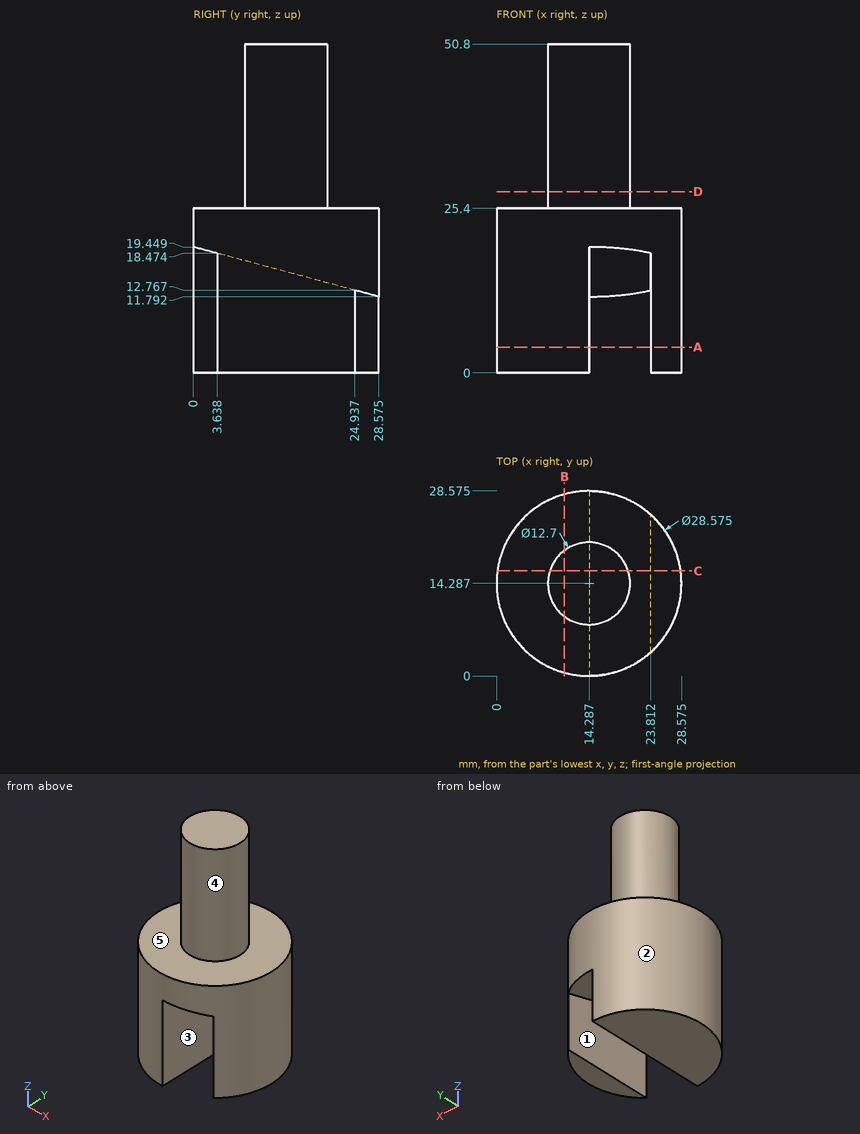
Geometry: see drawing. Coordinates: mm, zero at the bounding-box minimum. A direction names the side the tool comes from. Give positions to 0.01 mm unless a question says otherwise; leave off trailing zeros. Write each loop counter-clockwise with the first axis right and the second up, starting at its lowest first coordinate (ties: lowest second). Pieces come first, ordered by that corner, then holes. Notation, with made-up numbers: M 65,48 L 83,48 A16 ccw 83,68 Z; hole C -16.5,-21.5 d7. An arc over 180 degrees is marked long. Answer as a JSON object with one key per item and string values.
Q1. Cut plane C-C, the plane y = 16.25. Return the cut outline in (x, z) (1 decimal).
Geometry check:
{"outline": "M 0.1,0 L 14.3,0 L 14.3,15.1 L 23.8,15.1 L 23.8,0 L 28.4,0 L 28.4,25.4 L 20.3,25.4 L 20.3,50.8 L 8.2,50.8 L 8.2,25.4 L 0.1,25.4 Z"}
Q2. Access query for the marked faces 1 and 2. Directions: +Z, -Z, +X, -X, +Y, -Y. A direction counts if a zero-diameter tool reaches every point of the face in a straight line with its end or side. Return the directions, or none.
Geometry check:
{"face 1": "-Z, -Y", "face 2": "+Z, -Z"}
Q3. Ray query, line 1 along Z through (x, y) = (5, 14.75); line 2 along X through (y, z) = (10, 15.5) (1 decimal); line 3 along X through (y, z) = (9, 30) (1 decimal). Return the intervals inside material, ascending.
Geometry check:
{"line 1": "z = 0 to 25.4", "line 2": "x = 0.7 to 14.3, 23.8 to 27.9", "line 3": "x = 10.8 to 17.8"}
Q4. Cut plane B-B, the plane x = 10.5. Return the cut outline in (y, z) (1 decimal).
Geometry check:
{"outline": "M 0.5,0 L 28.1,0 L 28.1,25.4 L 19.4,25.4 L 19.4,50.8 L 9.2,50.8 L 9.2,25.4 L 0.5,25.4 Z"}
Q5. Mould query, pull axis X, two halves, no side actions, for the marked faces 3, 4 and 5. Classes: +X half, -X half, draft (parallel to the pull), parting line (faces both ways), or undercut.
Geometry check:
{"face 3": "undercut", "face 4": "parting line", "face 5": "draft"}
Q6. Cut plane A-A, the plane z = 4. Return the cut outline in (x, y) (1 decimal).
Geometry check:
{"outline": "M 14.3,0 L 14.3,28.6 A14.3 ccw Z; M 23.8,3.6 A14.3 ccw 23.8,24.9 Z"}
Q7. Cut plane D-D, the plane z = 28. Return the cut outline in (x, y).
Geometry check:
{"outline": "C 14.29,14.29 d12.7"}
Q8. Contact query for flat-ended pins moving along their axis: P1, Ø1, axis at x = 18, y = 7.5, coming from the +Z side; P2, Ø2, axis at y = 18.5, z = 25.5, coming from the +X side; P3, Ø10, axis at x = 10, z = 29.5, coming from the +Y side. Output: stop coordinate, or through.
Geometry check:
{"P1": "stops at z = 25.4", "P2": "stops at x = 28.21", "P3": "stops at y = 28.5"}
